Read the model definition and answer for the solid it produces. Units are mm, in the model's axes. A direction names the side the tool comes from. Coordinates: 2 decimals unless noted, no trailing zeros. Write each loop counter-clockwise with the first axis right and the second up, starting at its lowest first coordinate (ties: lowest second). Pieces come first, ordered by that corner, then holes. Notation, with made-up numbers: (-15.75, 67) -> (34.25, 67) arc R25 cw to (34.25, 86) -> close; hole circle Ø7 at (-6, 77.5). An arc over 180 degrees is marked (long way). Use CSV: the item, a comma, the result in double quotes.
Autodesk Fusion 360 part; units mm, degrees
sketch "Sketch1" plane through (0, 0, 0) normal (0, 0, 1) x (1, 0, 0) in component "Exercise3"
  circle A0 centre (0, 0) radius 10
  line L0 (0, 0) -> (30, 0) construction
  line L1 (0.1031, 19.9997) -> (30.1031, 19.9997)
  line L2 (0.1031, -19.9997) -> (30.1031, -19.9997)
  line L3 (30.1031, 19.9997) -> (30.1031, -20.0003)
  arc A1 (0.1031, 19.9997) -> (0.1031, -19.9997) centre (0, 0) ccw
  line L4 (20.1031, 19.9997) -> (20.1031, -19.9997)
  dimension "d1" = 20
  dimension "d2" = 40
  dimension "d3" = 30
  dimension "d4" = 30
  dimension "d5" = 30
  dimension "d6" = 40
  dimension "d7" = 10
extrude "Extrude1" add sketch "Sketch1" along normal blind 10 contours L1 L2 A1 L4 in component "Exercise3"
extrude "Extrude2" add sketch "Sketch1" along normal blind 50.06 contours L1 L2 L3 L4 in component "Exercise3"
fillet "Fillet1" radius 10 1 edges at (30.1031, 0, 0) in component "Exercise3"
sketch "Sketch2" plane through (0, 0, 50.06) normal (0, 0, 1) x (-1, 0, 0) in component "Exercise3"
  line L0 (-30.1031, -19.9997) -> (-20.1031, -19.9997)
  line L1 (-20.1031, -19.9997) -> (-20.1031, 19.9997)
  line L2 (-20.1031, 19.9997) -> (-30.1031, 19.9997)
  line L3 (-30.1031, 19.9997) -> (-30.1031, -19.9997)
  line L4 (-30.1031, 0) -> (0, 0) construction
  line L5 (-30.1031, -19.9997) -> (-0.1031, -19.9997)
  line L6 (-0.1031, -19.9997) -> (-0.1031, 19.9997)
  line L7 (-0.1031, 19.9997) -> (-30.1031, 19.9997)
  line L8 (-30.1031, 19.9997) -> (-30.1031, -19.9997)
  dimension "d13" = 30
extrude "Extrude3" add sketch "Sketch2" against normal blind 10 contours L1 L5 L6 L7 in component "Exercise3"
fillet "Fillet2" radius 10 2 edges at (0.1031, -19.9997, 45.06) (0.1031, 19.9997, 45.06) in component "Exercise3"
fillet "Fillet3" radius 10 1 edges at (20.1031, 0, 10) in component "Exercise3"
component "Exercise3" placed x (1, 0, 0) y (0, 1, 0) z (0, 0, 1) at (0, 0, 0)
1. A cutting plane is placed at B-B (x = -5). Give the vertices of the cut face in (y, z), and give its area (3 significant figures).
Solutions:
outline,"(-19.36, 0) -> (-8.66, 0) -> (-8.66, 10) -> (-19.36, 10) -> close; (8.66, 0) -> (19.36, 0) -> (19.36, 10) -> (8.66, 10) -> close"
area,"214 mm^2"
2. For a pull along Z with two mould halves and no side action, classify faces 4 (the cylindrical face through (2.95, 16.99, 44.99)), 5 (the flat face through (-12, 0, 10)), 6 (the flat face through (15, 0, 50.06)) as pulls with the +Z half, pulls with the -Z half, needs draft (parallel to the pull), parting line crosses it, or undercut.
Solutions:
face 4,"needs draft"
face 5,"undercut"
face 6,"pulls with the +Z half"
3. Each of these flat-tipped pins is pushed along its axis until it touches: pin 1 Ø22 at (y, z) = (0.5, 26.5) entering from -X; pin 2 Ø12 at (y, z) = (3.5, 24.5) entering from -X; pin 3 Ø8 at (y, z) = (1.5, 38.5) entering from -X. Where does it stop, or does it pass through?
Solutions:
pin 1,"stops at x = 19.03"
pin 2,"stops at x = 19.99"
pin 3,"stops at x = 0.1"
4. Find the intervals of material crossed by line 1 along Y through (x, z) = (0, 2); line 2 along Z through (x, y) = (-7, 10.5); line 3 along X through (y, z) = (-1, 20.5), in increasing order.
Solutions:
line 1,"y = -20 to -10, 10 to 20"
line 2,"z = 0 to 10"
line 3,"x = 20.1 to 30.1"
5. A tool of negligible diameter and unlimited length cuts with its end or side. For faces 1 (the cylindrical face through (-2.17, 9.76, 4.93)), 2 (the flat face through (10, 0, 40.06)), 3 (the cylindrical face through (3.11, -17.15, 44.99)), from which of +Z, -Z, +X, -X, +Y, -Y can it reach the whole face along a straight path? Write none if from no direction.
Solutions:
face 1,"-Z"
face 2,"-X, +Y, -Y"
face 3,"+Z, -X, -Y"
6. A cutting plane is placed at D-D (y = -13). Give the vertices of the cut face in (x, z), and give its area (3 significant figures).
Solutions:
outline,"(-15.2, 0) -> (20.1, 0) arc R10 ccw to (30.1, 10) -> (30.1, 50.06) -> (0.56, 50.06) -> (0.56, 40.06) -> (20.1, 40.06) -> (20.1, 20) arc R10 cw to (10.1, 10) -> (-15.2, 10) -> close"
area,"1,050 mm^2"
7. A cutting plane is placed at A-A (y = 0). Give the vertices of the cut face in (x, z).
Solutions:
outline,"(-20, 0) -> (-10, 0) -> (-10, 10) -> (-20, 10) -> close; (0.1, 40.06) -> (20.1, 40.06) -> (20.1, 20) arc R10 cw to (10.1, 10) -> (10, 10) -> (10, 0) -> (20.1, 0) arc R10 ccw to (30.1, 10) -> (30.1, 50.06) -> (0.1, 50.06) -> close"
8. A cutting plane is placed at C-C (x = 4.5). Give the vertices of the cut face in (y, z), and give its area (3 significant figures).
Solutions:
outline,"(-20, 0) -> (-8.93, 0) -> (-8.93, 10) -> (-20, 10) -> close; (-18.28, 40.06) -> (18.28, 40.06) -> (18.28, 50.06) -> (-18.28, 50.06) -> close; (8.93, 0) -> (20, 0) -> (20, 10) -> (8.93, 10) -> close"
area,"587 mm^2"
